Design review of the part shown in the three views and the two pictorial views. Dimensions are in mm from the part's minimum x, y and z. Give positions to 0.01 mm unless a question says otherwise; leave off trailing zeros. Loops run counter-clockwise (first coordinate to the right, second up) from the corner with the lowest first, then second, coordinate; pieces in that order, holes last. Notation, with made-up numbers: (48.25, 53) -> (91.25, 53) arc R16 ccw to (91.25, 65) -> close; hole circle Ø2 at (72, -35). An arc over 180 degrees is marked (long way). Use CSV: the item, a comma, the result in double quotes. Start each with the question number.
Item 1: We need section D-D (z = 22). State the section outline as (x, y) points, plus the area to 3 significant figures.
Item 2: We need section B-B (y = 1.3). State the section outline as (x, z) points (1 decimal).
Item 3: We need section A-A (z = 2.3). State the section outline as (x, y) points, plus the area to 3 significant figures.
Item 4: Wall thickness on line 1 along Z through (x, y) = (16, 0.8); line 2 along X through (y, z) = (0.85, 22); line 3 along X through (y, z) = (0.85, 22.25): over which ranges is each line inside the solid? List them lowest first. Write a range as from..to.
Item 5: We need section C-C (x = 12.5). State the section outline as (y, z) points.
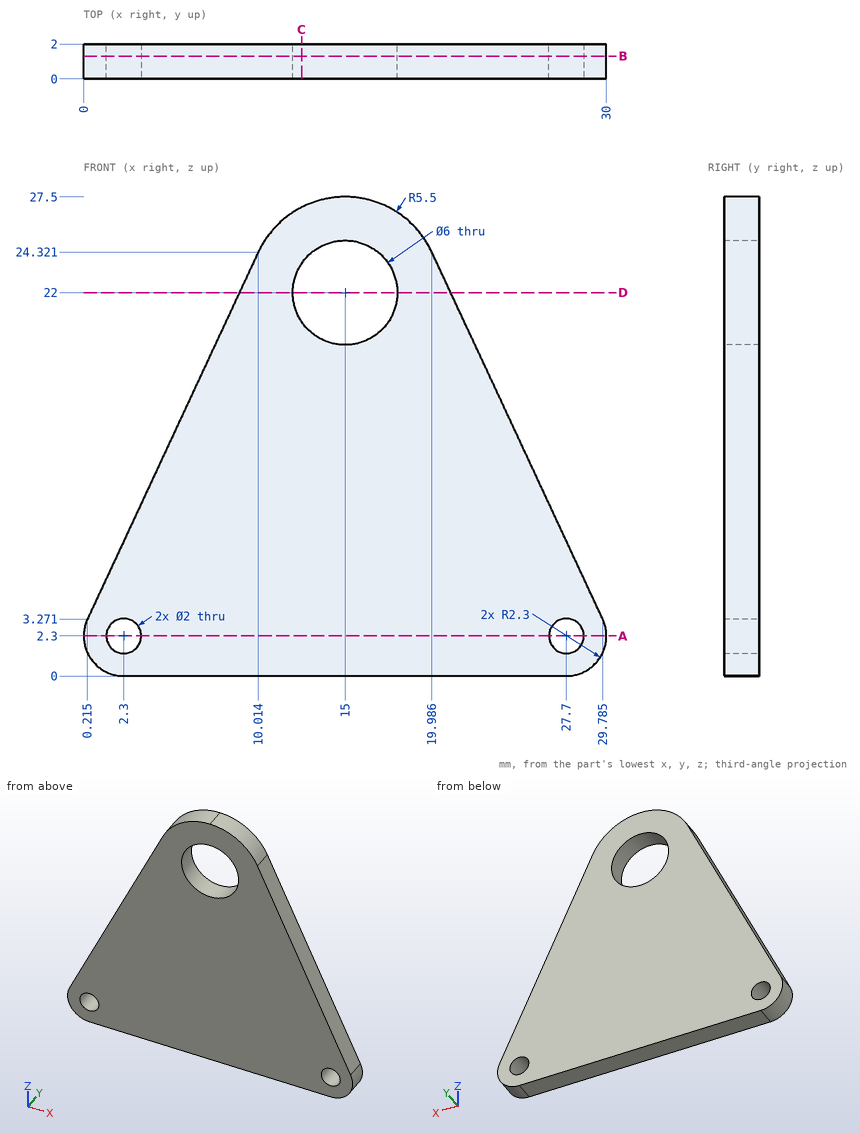
Results found:
1,outline,"(8.93, 0) -> (12, 0) -> (12, 2) -> (8.93, 2) -> close; (18, 0) -> (21.07, 0) -> (21.07, 2) -> (18, 2) -> close"
1,area,"12.3 mm²"
2,outline,"(0.2, 3.3) arc R2.3 ccw to (2.3, 0) -> (27.7, 0) arc R2.3 ccw to (29.8, 3.3) -> (20, 24.3) arc R5.5 ccw to (10, 24.3) -> close; hole circle Ø2 at (2.3, 2.3); hole circle Ø6 at (15, 22); hole circle Ø2 at (27.7, 2.3)"
3,outline,"(0, 0) -> (1.3, 0) -> (1.3, 2) -> (0, 2) -> close; (3.3, 0) -> (26.7, 0) -> (26.7, 2) -> (3.3, 2) -> close; (28.7, 0) -> (30, 0) -> (30, 2) -> (28.7, 2) -> close"
3,area,"52.0 mm²"
4,line 1,"0..19.17, 24.83..27.41"
4,line 2,"8.93..12, 18..21.07"
4,line 3,"9.05..12.01, 17.99..20.95"
5,outline,"(0, 0) -> (2, 0) -> (2, 20.34) -> (0, 20.34) -> close; (0, 23.66) -> (2, 23.66) -> (2, 26.9) -> (0, 26.9) -> close"
